Can you work these out from the model? Positions are in its coordinate system, mm. Face numbers are marked on the shaded views. A direction names the side the tool comes from. Round coordinates to 2 decimals unless told otherwise and drop trailing zeros. Loops run counter-clockwise (first coordinate to the right, second up) from the corner with the lowest first, then second, coordinate; pieces in that order, holes last. Notation, with made-up numbers: (-25, 15) -> (18, 15) arc R24 cw to (18, 51) -> close; hole circle Ø11 at (23.25, 57). An arc over 180 degrees is marked (long way). Use a Markdown table: item, result.
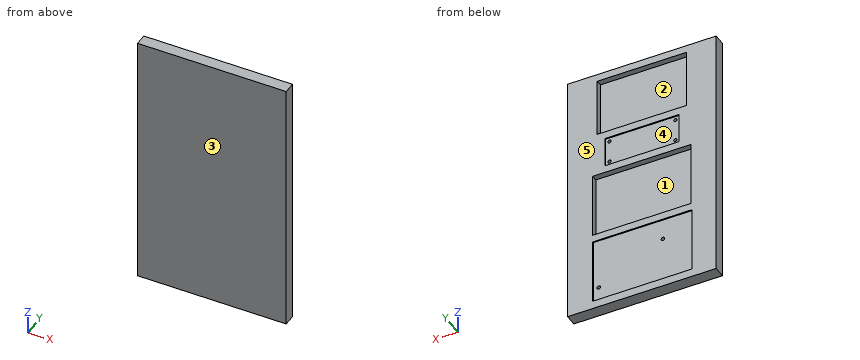
Autodesk Inventor part; units mm, degrees
ref_plane "YZ Plane" through (0, 0, 0) normal (1, 0, 0) x (0, 1, 0)
ref_plane "XZ Plane" through (0, 0, 0) normal (0, 1, 0) x (-1, 0, 0)
ref_plane "XY Plane" through (0, 0, 0) normal (0, 0, 1) x (1, 0, 0)
sketch "Sketch1" plane through (0, 0, 0) normal (0, 1, 0) x (-1, 0, 0)
  line L0 (0, 0) -> (-127, 0)
  line L1 (-127, 0) -> (-127, -222.25)
  line L2 (-127, -222.25) -> (0, -222.25)
  line L3 (0, -222.25) -> (0, 0)
  line L4 (0, 0) -> (-25.4, 0)
  line L5 (-127, 0) -> (-101.6, 0)
  line L6 (-25.4, 0) -> (-25.4, -6.35)
  line L7 (-101.6, 0) -> (-101.6, -6.35)
  line L8 (-25.4, -6.35) -> (-101.6, -6.35)
  line L9 (-101.6, -6.35) -> (-101.6, -57.15)
  line L10 (-101.6, -57.15) -> (-25.4, -57.15)
  line L11 (-25.4, -57.15) -> (-25.4, -6.35)
  dimension "d0" = 222.25
  dimension "d1" = 127
  dimension "d2" = 25.4
  dimension "d3" = 25.4
  dimension "d4" = 6.35
  dimension "d5" = 6.35
  dimension "d6" = 50.8
extrude "Extrusion1" add sketch "Sketch1" along normal blind 10.16
sketch "Sketch3" plane through (0, 10.16, 0) normal (0, 1, 0) x (1, 0, 0)
  line L0 (0, 0) -> (25.4, 0)
  line L1 (0, 0) -> (127, 0)
  line L2 (25.4, 0) -> (25.4, 6.35)
  line L3 (127, 0) -> (101.6, 0)
  line L4 (101.6, 0) -> (101.6, 6.35)
  line L5 (25.4, 6.35) -> (101.6, 6.35)
  line L6 (101.6, 6.35) -> (101.6, 57.15)
  line L7 (101.6, 57.15) -> (25.4, 57.15)
  line L8 (25.4, 57.15) -> (25.4, 6.35)
  line L9 (0, 222.25) -> (0, 0)
  line L10 (0, 57.15) -> (31.9532, 57.15)
  line L11 (127, 57.15) -> (95.0468, 57.15)
  line L12 (31.9532, 57.15) -> (31.9532, 63.5)
  line L13 (95.0468, 57.15) -> (95.0468, 63.5)
  line L14 (31.9532, 63.5) -> (95.0468, 63.5)
  line L15 (95.0468, 63.5) -> (95.0468, 89.4842)
  line L16 (95.0468, 89.4842) -> (31.9532, 89.4842)
  line L17 (31.9532, 89.4842) -> (31.9532, 63.5)
  line L18 (31.9532, 63.5) -> (31.9532, 66.929)
  line L19 (31.9532, 66.929) -> (35.3822, 66.929)
  line L20 (31.9532, 89.4842) -> (31.9532, 86.0552)
  line L21 (31.9532, 86.0552) -> (35.3822, 86.0552)
  line L22 (95.0468, 63.5) -> (95.0468, 66.929)
  line L23 (95.0468, 66.929) -> (91.6178, 66.929)
  line L24 (95.0468, 89.4842) -> (95.0468, 86.0552)
  line L25 (95.0468, 86.0552) -> (91.6178, 86.0552)
  circle A0 centre (91.6178, 66.929) radius 1.4478
  circle A1 centre (91.6178, 86.0552) radius 1.4478
  circle A2 centre (35.3822, 66.929) radius 1.4478
  circle A3 centre (35.3822, 86.0552) radius 1.4478
  line L26 (0, 89.4842) -> (21.463, 89.4842)
  line L27 (127, 0) -> (127, 222.25)
  line L28 (127, 89.4842) -> (105.537, 89.4842)
  line L29 (21.463, 89.4842) -> (21.463, 95.8342)
  line L30 (105.537, 89.4842) -> (105.537, 95.8342)
  line L31 (21.463, 95.8342) -> (105.537, 95.8342)
  line L32 (105.537, 95.8342) -> (105.537, 152.2222)
  line L33 (105.537, 152.2222) -> (21.463, 152.2222)
  line L34 (21.463, 152.2222) -> (21.463, 95.8342)
  line L35 (0, 152.2222) -> (20.7518, 152.2222)
  line L36 (127, 152.2222) -> (106.2482, 152.2222)
  line L37 (106.2482, 152.2222) -> (106.2482, 158.5722)
  line L38 (20.7518, 152.2222) -> (20.7518, 158.5722)
  line L39 (20.7518, 158.5722) -> (105.537, 158.5722)
  line L40 (105.537, 158.5722) -> (105.537, 215.2904)
  line L41 (105.537, 215.2904) -> (20.7518, 215.2904)
  line L42 (20.7518, 215.2904) -> (20.7518, 158.5722)
  line L43 (20.7518, 158.5722) -> (20.7518, 176.5554)
  line L44 (20.7518, 176.5554) -> (46.0502, 176.5554)
  line L45 (105.537, 215.2904) -> (105.537, 203.0984)
  line L46 (105.537, 203.0984) -> (100.9142, 203.0984)
  circle A4 centre (46.0502, 176.5554) radius 1.5494
  circle A5 centre (100.9142, 203.0984) radius 1.5494
  dimension "d15" = 25.4
  dimension "d16" = 6.35
  dimension "d17" = 25.4
  dimension "d18" = 6.35
  dimension "d19" = 50.8
  dimension "d20" = 31.9532
  dimension "d21" = 31.9532
  dimension "d22" = 6.35
  dimension "d23" = 25.9842
  dimension "d24" = 3.429
  dimension "d25" = 3.429
  dimension "d26" = 3.429
  dimension "d27" = 3.429
  dimension "d28" = 2.8956
  dimension "d29" = 2.8956
  dimension "d30" = 2.8956
  dimension "d31" = 2.8956
  dimension "d32" = 21.463
  dimension "d33" = 21.463
  dimension "d34" = 6.35
  dimension "d35" = 6.35
  dimension "d36" = 56.388
  dimension "d37" = 20.7518
  dimension "d38" = 20.7518
  dimension "d39" = 6.35
  dimension "d40" = 56.7182
  dimension "d41" = 17.9832
  dimension "d42" = 25.2984
  dimension "d43" = 12.192
  dimension "d44" = 4.6228
  dimension "d45" = 3.0988
  dimension "d46" = 3.0988
sketch "Sketch4" plane through (0, 10.16, 0) normal (0, 1, 0) x (1, 0, 0)
  circle A0 centre (91.6178, 66.929) radius 1.4478
  circle A1 centre (91.6178, 86.0552) radius 1.4478
  circle A2 centre (35.3822, 66.929) radius 1.4478
  circle A3 centre (35.3822, 86.0552) radius 1.4478
  circle A4 centre (46.0502, 176.5554) radius 1.5494
  circle A5 centre (100.9142, 203.0984) radius 1.5494
  point P0 (0, 0)
  dimension "d47" = 2.8956
  dimension "d48" = 2.8956
  dimension "d49" = 2.8956
  dimension "d50" = 2.8956
  dimension "d51" = 3.0988
  dimension "d52" = 3.0988
extrude "Extrusion2" cut sketch "Sketch3" against normal blind 5.08 contours L8 L7 L6 L5 | L34 L33 L32 L31
sketch "Sketch5" plane through (0, 10.16, 0) normal (0, 1, 0) x (1, 0, 0)
  line L0 (0, 0) -> (25.4, 0)
  line L1 (0, 0) -> (127, 0)
  line L2 (25.4, 0) -> (25.4, 6.35)
  line L3 (127, 0) -> (101.6, 0)
  line L4 (101.6, 0) -> (101.6, 6.35)
  line L5 (25.4, 6.35) -> (101.6, 6.35)
  line L6 (101.6, 6.35) -> (101.6, 57.15)
  line L7 (101.6, 57.15) -> (25.4, 57.15)
  line L8 (25.4, 57.15) -> (25.4, 6.35)
  line L9 (0, 222.25) -> (0, 0)
  line L10 (0, 57.15) -> (31.9532, 57.15)
  line L11 (127, 57.15) -> (95.0468, 57.15)
  line L12 (31.9532, 57.15) -> (31.9532, 63.5)
  line L13 (95.0468, 57.15) -> (95.0468, 63.5)
  line L14 (31.9532, 63.5) -> (95.0468, 63.5)
  line L15 (95.0468, 63.5) -> (95.0468, 89.4842)
  line L16 (95.0468, 89.4842) -> (31.9532, 89.4842)
  line L17 (31.9532, 89.4842) -> (31.9532, 63.5)
  line L18 (31.9532, 63.5) -> (31.9532, 66.929)
  line L19 (31.9532, 66.929) -> (35.3822, 66.929)
  line L20 (31.9532, 89.4842) -> (31.9532, 86.0552)
  line L21 (31.9532, 86.0552) -> (35.3822, 86.0552)
  line L22 (95.0468, 63.5) -> (95.0468, 66.929)
  line L23 (95.0468, 66.929) -> (91.6178, 66.929)
  line L24 (95.0468, 89.4842) -> (95.0468, 86.0552)
  line L25 (95.0468, 86.0552) -> (91.6178, 86.0552)
  circle A0 centre (91.6178, 66.929) radius 1.4478
  circle A1 centre (91.6178, 86.0552) radius 1.4478
  circle A2 centre (35.3822, 66.929) radius 1.4478
  circle A3 centre (35.3822, 86.0552) radius 1.4478
  line L26 (0, 89.4842) -> (21.463, 89.4842)
  line L27 (127, 0) -> (127, 222.25)
  line L28 (127, 89.4842) -> (105.537, 89.4842)
  line L29 (21.463, 89.4842) -> (21.463, 95.8342)
  line L30 (105.537, 89.4842) -> (105.537, 95.8342)
  line L31 (21.463, 95.8342) -> (105.537, 95.8342)
  line L32 (105.537, 95.8342) -> (105.537, 152.2222)
  line L33 (105.537, 152.2222) -> (21.463, 152.2222)
  line L34 (21.463, 152.2222) -> (21.463, 95.8342)
  line L35 (0, 152.2222) -> (20.7518, 152.2222)
  line L36 (127, 152.2222) -> (106.2482, 152.2222)
  line L37 (106.2482, 152.2222) -> (106.2482, 158.5722)
  line L38 (20.7518, 152.2222) -> (20.7518, 158.5722)
  line L39 (20.7518, 158.5722) -> (105.537, 158.5722)
  line L40 (105.537, 158.5722) -> (105.537, 215.2904)
  line L41 (105.537, 215.2904) -> (20.7518, 215.2904)
  line L42 (20.7518, 215.2904) -> (20.7518, 158.5722)
  line L43 (20.7518, 158.5722) -> (20.7518, 176.5554)
  line L44 (20.7518, 176.5554) -> (46.0502, 176.5554)
  line L45 (105.537, 215.2904) -> (105.537, 203.0984)
  line L46 (105.537, 203.0984) -> (100.9142, 203.0984)
  circle A4 centre (46.0502, 176.5554) radius 1.5494
  circle A5 centre (100.9142, 203.0984) radius 1.5494
  dimension "d55" = 25.4
  dimension "d56" = 6.35
  dimension "d57" = 25.4
  dimension "d58" = 6.35
  dimension "d59" = 50.8
  dimension "d60" = 31.9532
  dimension "d61" = 31.9532
  dimension "d62" = 6.35
  dimension "d63" = 25.9842
  dimension "d64" = 3.429
  dimension "d65" = 3.429
  dimension "d66" = 3.429
  dimension "d67" = 3.429
  dimension "d68" = 2.8956
  dimension "d69" = 2.8956
  dimension "d70" = 2.8956
  dimension "d71" = 2.8956
  dimension "d72" = 21.463
  dimension "d73" = 21.463
  dimension "d74" = 6.35
  dimension "d75" = 6.35
  dimension "d76" = 56.388
  dimension "d77" = 20.7518
  dimension "d78" = 20.7518
  dimension "d79" = 6.35
  dimension "d80" = 56.7182
  dimension "d81" = 17.9832
  dimension "d82" = 25.2984
  dimension "d83" = 12.192
  dimension "d84" = 4.6228
  dimension "d85" = 3.0988
  dimension "d86" = 3.0988
extrude "Extrusion3" cut sketch "Sketch5" against normal blind 1.016 contours L42 L41 L40 L39 | L17 L16 L15 L14
extrude "Extrusion4" cut sketch "Sketch4" against normal blind 7.62
properties part number "base embed"
1. Which directions (+Z, -Z, +X, -X, +Y, -Y) give clear straight access to the entire face, cutting with the end or side of a thin tool? Please do the marked faces 4 and 5.
Answer sheet:
| item | result |
|---|---|
| face 4 | +Y |
| face 5 | +Z, -Z, +X, -X, +Y |
2. Will this pin go through, and if not, where does the flat tip stop? pin 1 Ø8 at (x, z) = (49, -80.5) entering from +Y.
Answer sheet:
| item | result |
|---|---|
| pin 1 | stops at y = 9.14 |
3. I want a section at D-D (z = -40). Please give me the cut outline in (x, y).
Answer sheet:
| item | result |
|---|---|
| outline | (0, 0) -> (127, 0) -> (127, 10.16) -> (101.6, 10.16) -> (101.6, 5.08) -> (25.4, 5.08) -> (25.4, 10.16) -> (0, 10.16) -> close |
4. If we mould it in two halves opening along X, with no side actions, what happens to the marked faces 1, 2 and 3? For each: +X half, -X half, draft (parallel to the pull), parting line (faces both ways), or undercut.
Answer sheet:
| item | result |
|---|---|
| face 1 | undercut |
| face 2 | undercut |
| face 3 | draft |
5. I want a section at A-A (z = -142.5). Please give me the cut outline in (x, y), plus the area to 3 significant figures.
Answer sheet:
| item | result |
|---|---|
| outline | (0, 0) -> (127, 0) -> (127, 10.16) -> (105.54, 10.16) -> (105.54, 5.08) -> (21.46, 5.08) -> (21.46, 10.16) -> (0, 10.16) -> close |
| area | 863 mm² |
6. I want a section at C-C (y = 7.25). State how many separate pieces and enclosed holes the cut face has, plus the area to 3 significant figures.
Answer sheet:
| item | result |
|---|---|
| separate pieces | 1 |
| enclosed holes | 8 |
| area | 19,600 mm² |
7. I want a section at B-B (x = 69). Please give me the cut outline in (y, z).
Answer sheet:
| item | result |
|---|---|
| outline | (0, -222.25) -> (10.16, -222.25) -> (10.16, -215.29) -> (9.14, -215.29) -> (9.14, -158.57) -> (10.16, -158.57) -> (10.16, -152.22) -> (5.08, -152.22) -> (5.08, -95.83) -> (10.16, -95.83) -> (10.16, -89.48) -> (9.14, -89.48) -> (9.14, -63.5) -> (10.16, -63.5) -> (10.16, -57.15) -> (5.08, -57.15) -> (5.08, -6.35) -> (10.16, -6.35) -> (10.16, 0) -> (0, 0) -> close |
8. I need wall thicknesses on line 1 (Z direction, x = 61.5, y = 9); line 2 (X direction, y = 7.5, z = -96); line 3 (X direction, y = 5.5, z = -19). Which ranges of each line are inside material? Lowest first, please.
Answer sheet:
| item | result |
|---|---|
| line 1 | z = -222.25 to -152.22, -95.83 to -57.15, -6.35 to 0 |
| line 2 | x = 0 to 21.46, 105.54 to 127 |
| line 3 | x = 0 to 25.4, 101.6 to 127 |
